Check sheet for the drawn part. Datum: minimum x, y, z corner. Units: mm. Coordinates: 2 decimals unless noted, no trailing zeros. Order: outer loops, then holes, each group sorted by start corner. A loop starts at its lowest first (then second) coordinate and runs counter-clockwise, first axis right, second up.
Q1. Thickness scan on line 1 (Z direction, x = 20, y = 1.4); line 2 (Z direction, x = 102.5, y = 1.3); line 3 (X direction, y = 0.85, z = 42.5). Record the ranges inside material, lowest first.
Q2. Cross-section at B-B, the plane x = 20. Record the boundary of the cut face in (y, z), and give its area (3 significant figures).
Q3. Cross-section at A-A, the plane z = 42.5. Record the boundary of the cut face in (x, y), and give its area (3 significant figures).
Q4. Cross-section at C-C, the plane y = 2.7. Count the separate pieces of the cut face and the enclosed holes in it, and give its area (3 significant figures).
Q5. Cross-section at D-D, the plane z = 5. Record the boundary of the cut face in (x, y).
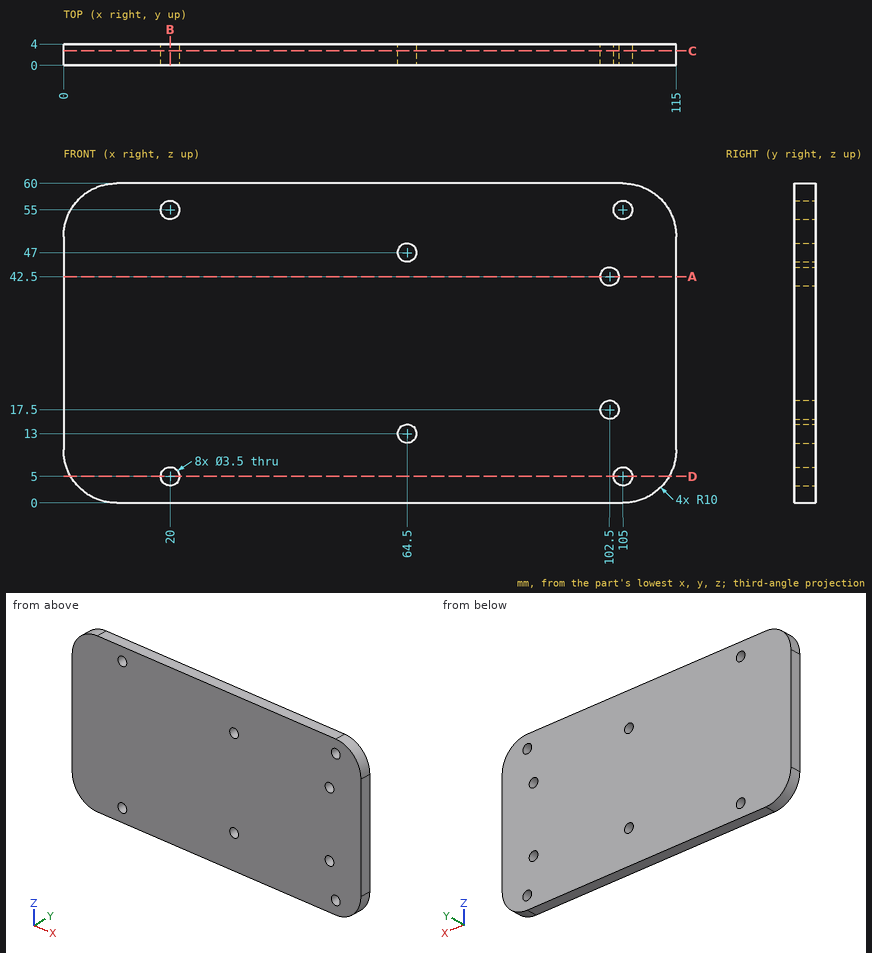
Check values:
1. line 1: z = 0 to 3.25, 6.75 to 53.25, 56.75 to 60
1. line 2: z = 0 to 15.75, 19.25 to 40.75, 44.25 to 60
1. line 3: x = 0 to 100.75, 104.25 to 115
2. outline: (0, 0) - (4, 0) - (4, 3.25) - (0, 3.25) - close; (0, 6.75) - (4, 6.75) - (4, 53.25) - (0, 53.25) - close; (0, 56.75) - (4, 56.75) - (4, 60) - (0, 60) - close
2. area: 212 mm2
3. outline: (0, 0) - (100.75, 0) - (100.75, 4) - (0, 4) - close; (104.25, 0) - (115, 0) - (115, 4) - (104.25, 4) - close
3. area: 446 mm2
4. separate pieces: 1
4. enclosed holes: 8
4. area: 6,740 mm2
5. outline: (1.34, 0) - (18.25, 0) - (18.25, 4) - (1.34, 4) - close; (21.75, 0) - (103.25, 0) - (103.25, 4) - (21.75, 4) - close; (106.75, 0) - (113.66, 0) - (113.66, 4) - (106.75, 4) - close
